```python
from build123d import *

# Parameters (mm, degrees)
BOSS_EXTRUDE1_DEPTH = 12
BOSS_EXTRUDE2_START = 4
SKETCH2_W           = 10
SKETCH2_H           = 7.500000000000002
SKETCH2_R           = 1.65
BOSS_EXTRUDE2_DEPTH = 4
SKETCH3_W           = 10
SKETCH3_H           = 7.499999999999999
SKETCH3_R           = 1.6500000000000001
BOSS_EXTRUDE3_DEPTH = 4
SKETCH4_R           = 5.000000000000002
BOSS_EXTRUDE4_DEPTH = 26
CUT_EXTRUDE1_DEPTH  = 39.44801685392889
CUT_EXTRUDE2_DEPTH  = 41.277164746292655
VARFILLET1_START    = -5
VARFILLET1_DEPTH    = 22


with BuildPart() as part:
    # Sketch1 → Boss-Extrude1 (new body)
    with BuildSketch(Plane(origin=(0, 0, 0), x_dir=(1, 0, 0), z_dir=(0, 1, 0))):
        with BuildLine():
            Line((-5, 7.5), (-10, 7.499999999999999))
            Line((-10, 7.499999999999999), (-10, 6.009988028713897))
            ThreePointArc((-10, 6.009988028713897), (-9.937986363684939, 5.515813106068849), (-9.755791145828766, 5.052283767352735))
            Line((-9.755791145828766, 5.052283767352735), (-7.56852494834847, 1.0422957386388614))
            ThreePointArc((-7.56852494834847, 1.042295738638861), (-6.83366266323373, 0.2802022614966764), (-5.812733802519688, -8.9e-16))
            Line((-5.812733802519688, 0), (-5, 0))
            Line((-5, 0), (-5, 2.0999999999999996))
            ThreePointArc((-5.000000000000002, 2.0999999999999996), (-6.65, 3.7500000000000004), (-5, 5.3999999999999995))
            Line((-5, 5.3999999999999995), (-5, 7.5))
        make_face()
        with BuildLine():
            Line((0, 7.5), (-5, 7.5))
            Line((-5, 7.5), (-5, 5.3999999999999995))
            ThreePointArc((-5, 5.3999999999999995), (-3.8332738110421967, 4.916726188957803), (-3.35, 3.7499999999999996))
            ThreePointArc((-3.35, 3.749999999999999), (-3.833273811042198, 2.583273811042195), (-5.000000000000002, 2.0999999999999996))
            Line((-5, 2.0999999999999996), (-5, 0))
            Line((-5, 0), (-4.187266197480313, 0))
            ThreePointArc((-4.187266197480313, -8.9e-16), (-3.1663373367662704, 0.2802022614966755), (-2.4314750516515296, 1.0422957386388605))
            Line((-2.43147505165153, 1.0422957386388614), (-0.24420885417123472, 5.052283767352735))
            ThreePointArc((-0.24420885417123483, 5.052283767352735), (-0.06201363631506229, 5.515813106068849), (0, 6.009988028713897))
            Line((0, 6.009988028713897), (0, 7.5))
        make_face()
    extrude(amount=BOSS_EXTRUDE1_DEPTH)

    # Sketch2 → Boss-Extrude2 (add)
    with BuildSketch(Plane.XZ.offset(BOSS_EXTRUDE2_START)):
        with Locations((-5, -3.75)):
            Rectangle(SKETCH2_W, SKETCH2_H)
        with Locations(Location((-4.999999999999999, -3.75, 0), (0, 0, 270))):
            Circle(SKETCH2_R, mode=Mode.SUBTRACT)
    extrude(amount=-BOSS_EXTRUDE2_DEPTH)

    # Sketch3 → Boss-Extrude3 (add)
    with BuildSketch(Plane(origin=(0, 12, 0), x_dir=(1, 0, 0), z_dir=(0, 1, 0))):
        with Locations((-5, 3.7499999999999996)):
            Rectangle(SKETCH3_W, SKETCH3_H)
        with Locations(Location((-4.999999999999999, 3.7499999999999982, 0), (0, 0, 90))):
            Circle(SKETCH3_R, mode=Mode.SUBTRACT)
    extrude(amount=BOSS_EXTRUDE3_DEPTH)

    # Sketch4 → Boss-Extrude4 (add)
    with BuildSketch(Plane(origin=(-6.5e-16, 0, -7.5), x_dir=(-1, 0, 9e-17), z_dir=(-9e-17, 0, -1))):
        with Locations((5, 6)):
            Circle(SKETCH4_R)
    extrude(amount=BOSS_EXTRUDE4_DEPTH)

    # Sketch5 → Cut-Extrude1 (cut, through all)
    with BuildSketch(Plane(origin=(0, 0, 0), x_dir=(0, 0, -1), z_dir=(1, 0, 0))):
        Polygon((33.5, 11.000000000000002), (7.5, 11), (33.5, 7), align=None)
        Polygon((33.5, 0.9999999999999991), (33.5, 5), (7.5, 0.9999999999999991), align=None)
    extrude(amount=-CUT_EXTRUDE1_DEPTH, mode=Mode.SUBTRACT)

    # Sketch6 → Cut-Extrude2 (cut, through all)
    with BuildSketch(Plane(origin=(0, -4, 0), x_dir=(-1, 0, 0), z_dir=(0, -1, 0))):
        Polygon((3.47e-15, 7.5), (4.0000000000000036, 33.500000000000014), (3.6e-15, 33.500000000000014), align=None)
        Polygon((10.000000000000007, 33.500000000000014), (6.0000000000000036, 33.500000000000014), (10, 7.5), align=None)
    extrude(amount=-CUT_EXTRUDE2_DEPTH, mode=Mode.SUBTRACT)

    # VarFillet1: read off the stored shape, not the designer's step
    # VarFillet1 outline → VarFillet1 (cut)
    with BuildSketch(Plane(origin=(0, 0, 0), x_dir=(1, 0, 0), z_dir=(0, 1, 0)).offset(VARFILLET1_START)):
        with BuildLine():
            Line((0, 0), (0, 2))
            add(Edge.make_bspline(
                [(0, 2), (0, 0), (-2, 0)],
                knots=[0, 0, 0, 1, 1, 1], degree=2, weights=[1, 0.707106781186548, 1]))
            Line((-2, 0), (0, 0))
        make_face()
        with BuildLine():
            Line((-10, 0), (-8, 0))
            add(Edge.make_bspline(
                [(-8, 0), (-10, 0), (-10, 2)],
                knots=[0, 0, 0, 1, 1, 1], degree=2, weights=[1, 0.707106781186548, 1]))
            Line((-10, 2), (-10, 0))
        make_face()
    extrude(amount=VARFILLET1_DEPTH, mode=Mode.SUBTRACT)


solid = part.part
```
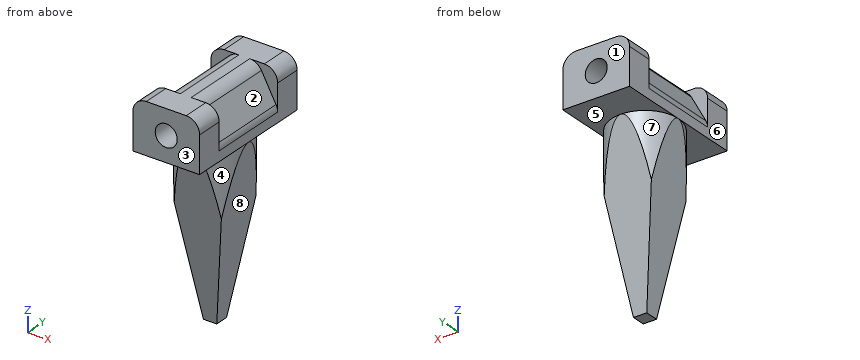
For this review, take the finished solid that the model builds, in its own axes (mm). Face numbers are marked on the shaded views. A direction names the side the tool comes from. Give positions to 0.01 mm unless a question says otherwise; leave off trailing zeros. Loops run counter-clockwise (first coordinate to the right, second up) from the corner with the lowest first, then second, coordinate; pieces in that order, holes last. Notation, with made-up numbers: M 15.25,7.5 L 61.25,7.5 A29 cw 61.25,27.5 Z; hole C 4.5,47.5 d1. An arc over 180 degrees is marked long. One line per item, written item: value. Start each with the question number.
Q1. Add section A-A (z = -3.75). Give the boundary of the cut face in (x, y).
Q2. Add section D-D (z = -28). Give the boundary of the cut face in (x, y), and give its area (3 significant figures).
Q3. Add section C-C (z = -11.5). Give the boundary of the cut face in (x, y), and give its area (4 significant figures).
Q4. Machinability: for the marked faces 4, 5, 6, 7 and 8, which of the approach directions +Z, -Z, +X, -X, +Y, -Y give a long, thin tool a straight path to every point of the face, cutting with its end or side? Answer none if there is none.
Q5. Draft analysis for pull direction Y (two halves, no side actions). For the marked faces 1, 2 and 3, state which applies: released by +Y, released by -Y, zero draft, split by the parting line, or undercut.
Q6. For L1, parallel to X at y = 6, z = -3.75; L2, parallel to X at y = 0.5, z = -4.5; L3, parallel to Z at x = -5.5, y = 6.75, list the stretches that pass through material, from the lowest coordinate up.
Q7. Clearance check with flat-ended pins moving along their axes: pin 1 Ø2 at (y, z) = (4.5, -26) entering from -X; pin 2 Ø1 at (y, z) = (7, -14.5) entering from -X; pin 3 Ø1 at (x, z) = (-2.5, -18.5) entering from -Y. State where each tip first meets the part, or that it passes through.
Reply:
1. outline: M -10,-4 L -6.65,-4 L -6.65,16 L -10,16 L -10,12 L -9.05,12 L -9.05,0 L -10,0 Z; M -3.35,-4 L 0,-4 L 0,0 L -0.95,0 L -0.95,12 L 0,12 L 0,16 L -3.35,16 Z
2. outline: M -6.85,4.15 L -3.15,4.15 L -3.15,7.85 L -6.85,7.85 Z
2. area: 13.6 mm²
3. outline: M -9.38,3.6 A5 ccw -7.4,1.62 L -2.6,1.62 A5 ccw -0.62,3.6 L -0.62,8.4 A5 ccw -2.6,10.38 L -7.4,10.38 A5 ccw -9.38,8.4 Z
3. area: 70.55 mm²
4. face 4: -Z, +X, -Y
4. face 5: -Z, +Y
4. face 6: +Z, -Z, -X, +Y, -Y
4. face 7: -Z, -X, +Y
4. face 8: -Z, +X, +Y, -Y
5. face 1: released by +Y
5. face 2: undercut
5. face 3: released by -Y
6. L1: -9.05 to -6.65, -3.35 to -0.95
6. L2: -9.45 to -6.47, -3.53 to -0.55
6. L3: -33.5 to -5.32, -2.18 to 0
7. pin 1: x = -7.31
7. pin 2: x = -9
7. pin 3: y = 2.62
